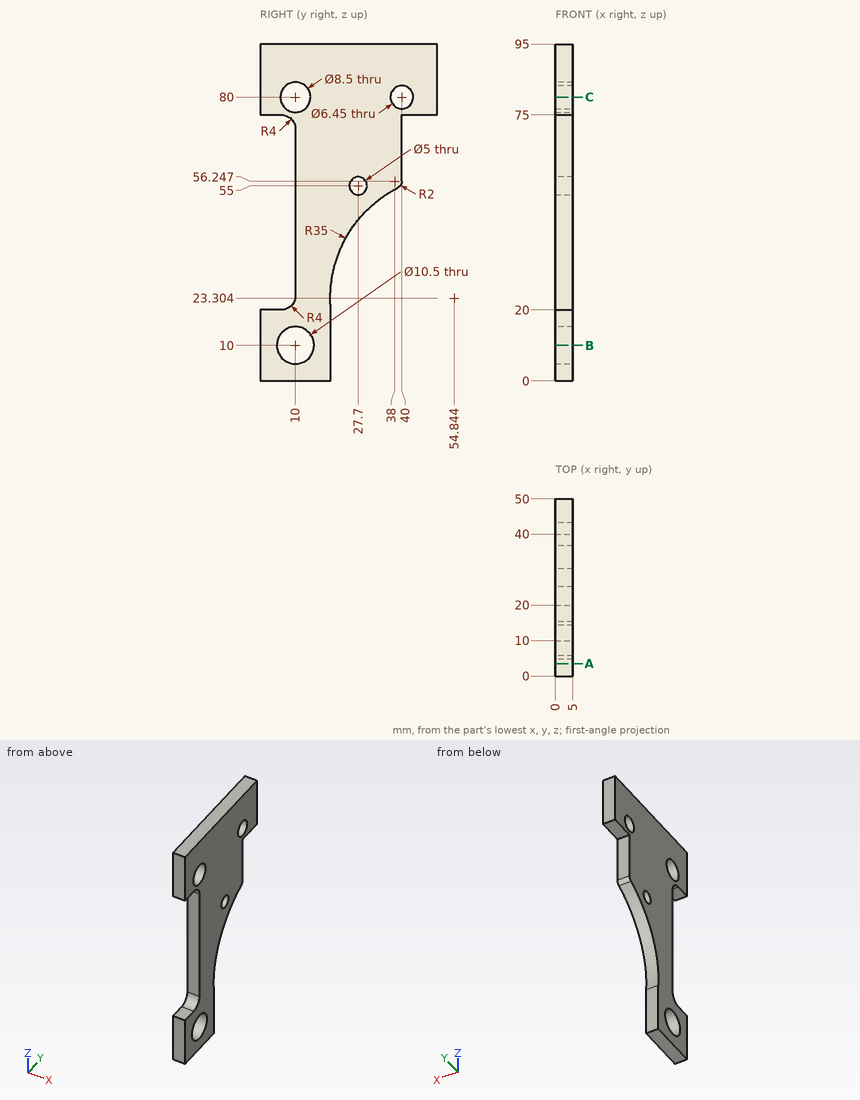
Study the drawing (mm; zero at the part's minimum x, y, z) and answer. Give positions to 0.01 mm unless a question says otherwise; leave off trailing zeros. Write each loop counter-clockwise with the first axis right and the second up, starting at its lowest first coordinate (ties: lowest second). Pieces come first, ordered by that corner, then holes. Notation, with made-up numbers: (-3, -35) -> (22, -35) arc R30 cw to (22, -3) -> close; hole circle Ø4 at (-33, -26.75). An arc over 180 degrees is marked (long way). Write item = value, one per line.
Q1. Section B-B on z = 10 is taken. Determine the outline of the cut face in (x, y).
Computed values:
outline = (0, 0) -> (5, 0) -> (5, 4.75) -> (0, 4.75) -> close; (0, 15.25) -> (5, 15.25) -> (5, 20) -> (0, 20) -> close
Q2. Section A-A on y = 3.5 is taken. Determine the outline of the cut face in (x, z), and give its area (3 significant figures).
Computed values:
outline = (0, 0) -> (5, 0) -> (5, 20) -> (0, 20) -> close; (0, 75) -> (5, 75) -> (5, 95) -> (0, 95) -> close
area = 200 mm^2
Q3. Section C-C on z = 80 is taken. State how many separate pieces and enclosed holes the cut face has, and give its area (3 significant figures).
Computed values:
separate_pieces = 3
enclosed_holes = 0
area = 175 mm^2
Q4. Flat-ended cylindrical pins translate along their axes: pin 1 Ø6 at (y, z) = (41, 56) entering from +X; pin 2 Ø5 at (y, z) = (10, 80) entering from +X (3 decimals); pin 3 Ø2.5 at (x, y) = (3.5, 44) entering from -Z; pin 4 Ø1.5 at (x, z) = (2.5, 59) entering from -Y. Find the tip coordinate at first contact, or state that the pin passes through.
Computed values:
pin_1 = 5
pin_2 = through
pin_3 = 75
pin_4 = 10
Q5. Consider line 1 along Z through (x, y) = (2.7, 4.5); line 2 along Y through (x, z) = (2, 10); line 3 along Y through (x, z) = (2.95, 81) (1 decimal). Determine where each line is inside the solid, lowest interval first.
Computed values:
line_1 = 0 to 20, 75 to 95
line_2 = 0 to 4.75, 15.25 to 20
line_3 = 0 to 5.9, 14.1 to 36.9, 43.1 to 50
